Study the drawing (mm; zero at the part's minimum x, y, z) and answer. Give positions to 0.01 mm unless a question says otherwise; leave off trailing zeros. Loops run counter-clockwise (first coordinate to the right, second up) from the corner with the lowest first, then second, coordinate; pieces in that order, holes last. Notation, with made-up numbers: M 83.25,-18.75 L 139.25,-18.75 A27 cw 139.25,3.25 Z; hole C 33.25,-28 d3. An arc over 180 degrees is marked long. Use one line per item in the form item = value. Start each with the question number.
1. The part is cut by section C-C (x = 97.5). Write down the section's boundary in (y, z).
2. The part is cut by section A-A (y = 40). Write down the section's boundary in (x, z), and give its area (3 significant figures).
3. The part is cut by section B-B (x = 134). Write down the section's boundary in (y, z).
4. The part is cut by section D-D (z = 11). Write down the section's boundary in (x, y), and give its area (3 significant figures).
5. Each of these flat-tipped pins is pushed along its axis until it touches: pin 1 Ø3 at (x, y) = (33.5, 64) entering from +Z; pin 2 Ø12 at (x, y) = (162.5, 18.5) entering from -Z (3 decimals); pin 3 Ø18 at (x, y) = (125, 40) entering from -Z. Where does it stop, or does it pass through?
6. The mould has two halves that part along X. Classify the marked faces 1, 2, 3 and 4: released by +X, released by -X, zero draft, split by the parting line, or undercut.
7. Straight lines are drawn through the part: line 1 (Z direction, x = 177, y = 40); line 2 (Y direction, x = 112, z = 6.5) (1 decimal). For each, find the intervals that lie inside material, in ascending order. Write a range as from..to.
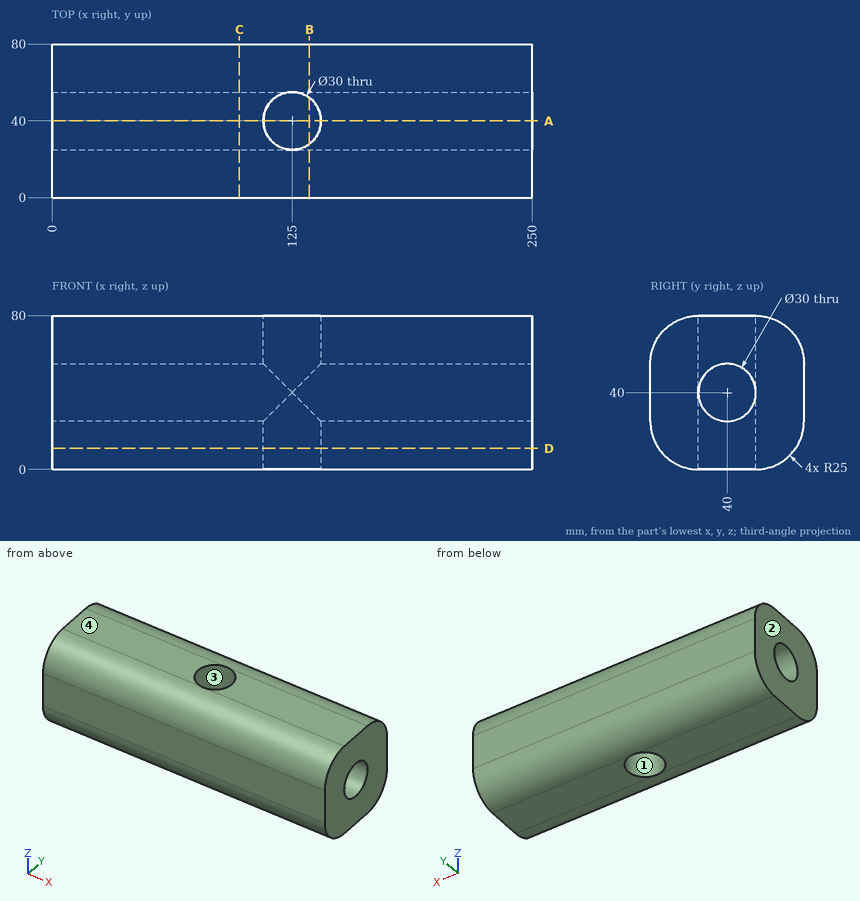
Derived:
q1.outline = M 0,25 A25 ccw 25,0 L 55,0 A25 ccw 80,25 L 80,55 A25 ccw 55,80 L 25,80 A25 ccw 0,55 Z; hole C 40,40 d30
q2.outline = M 0,0 L 110,0 L 110,25 L 0,25 Z; M 0,55 L 110,55 L 110,80 L 0,80 Z; M 140,0 L 250,0 L 250,25 L 140,25 Z; M 140,55 L 250,55 L 250,80 L 140,80 Z
q2.area = 11,000 mm2
q3.outline = M 0,25 A25 ccw 25,0 L 28,0 L 28,31 A15 cw 28,49 L 28,80 L 25,80 A25 ccw 0,55 Z; M 52,0 L 55,0 A25 ccw 80,25 L 80,55 A25 ccw 55,80 L 52,80 L 52,49 A15 cw 52,31 Z
q4.outline = M 0,4.29 L 250,4.29 L 250,75.71 L 0,75.71 Z; hole C 125,40 d30
q4.area = 17,100 mm2
q5.pin_1 = 78.85
q5.pin_2 = 0.005
q5.pin_3 = through
q6.face_1 = undercut
q6.face_2 = released by -X
q6.face_3 = undercut
q6.face_4 = zero draft
q7.line_1 = 0..25, 55..80
q7.line_2 = 8.2..32.5, 47.5..71.8
